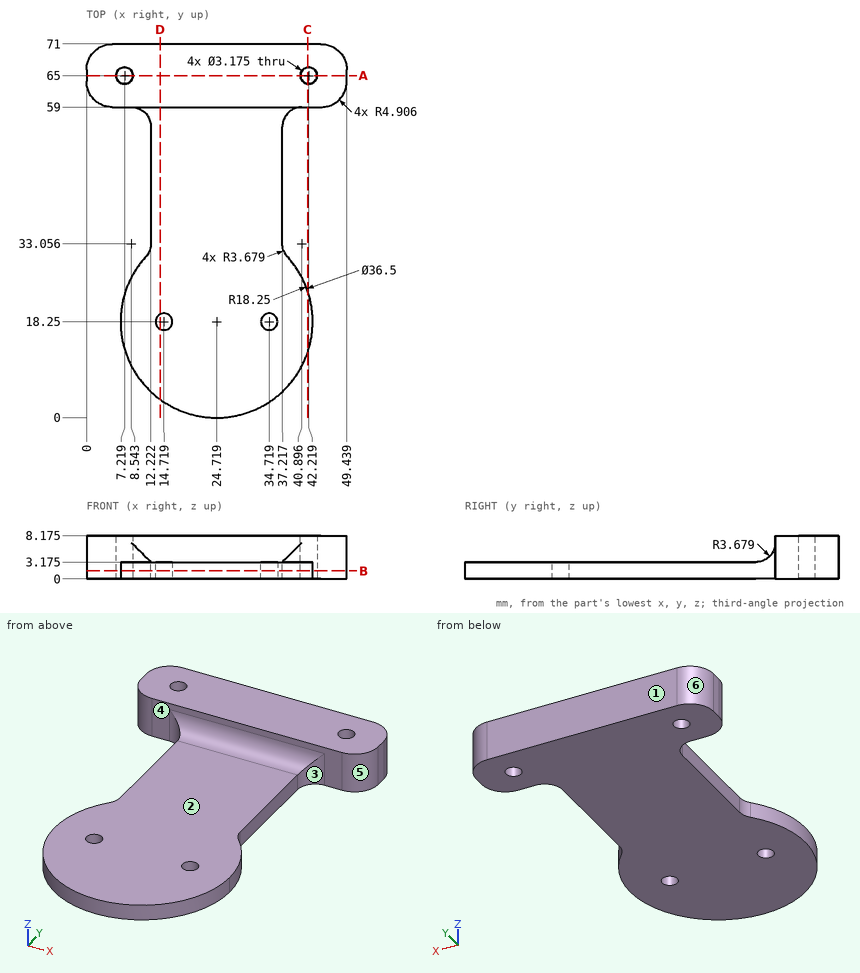
Here's the drawing with two shaded views (mm, measured from the low corner). I have some questions. A direction names the side the tool comes from. Round coordinates to 2 decimals unless told otherwise and drop trailing zeros. Loops run counter-clockwise (first coordinate to the right, second up) from the corner with the lowest first, then second, coordinate; pieces in that order, holes last. Notation, with made-up numbers: M -0.75,-12 L 25.25,-12 A15 ccw 25.25,16 Z; hole C -23.5,-35.5 d7. An arc over 180 degrees is marked long. Answer as a JSON object with one key per item and string values. Group by question number.
Q1. We'd pull the mould along Y, two halves only. Please class the marked faces 3, 4, 5 and 6: +Y half, -Y half, draft (parallel to the pull), parting line (faces both ways), or undercut.
Q2. Imagine slicing it at B-B, the plane z = 1.5. Count the separate pieces of the cut face and the enclosed holes in it, then the cut area to 3 significant figures.
Q3. Imagine slicing it at D-D, the plane x = 14. Please give me the cut outline in (y, z) (1 decimal).
Q4. Will these pins go through, and if not, where does the flat tip stop? pin 1 (3 mm diameter, centred on x = 42.22, y = 65, fed in from -Z); pin 2 (4 mm diameter, centred on y = 23.5, z = 4, fed in from -X); pin 3 (3.5 mm diameter, centred on x = 14.72, y = 18.25, fed in from +Z) (3 decimals); pin 4 (4 mm diameter, centred on x = 16, z = 3, fed in from -Y).
Q5. Please list where these lines run through material, in increasing order: L1, parallel to X at y = 18.25, z = 1.6; L2, parallel to X at y = 65, z = 4.75; L3, parallel to Y at x = 43.5, z = 2.75.
Q6. On a 3-axis mill with a long thin cutter (end or side, diameter ignored), from which of +Z, -Z, +X, -X, +Y, -Y can I reach the whole of each face in a straight line? I mean the marked faces 1 and 2. Say none if no direction works.
Q7. Imagine slicing it at C-C, the plane x = 42. Please give me the cut outline in (y, z) (1 decimal), then the cut area to 3 significant figures.
Q8. Imagine slicing it at A-A, the plane y = 65. Please give me the cut outline in (x, z) (1 decimal), then the cut area to 3 significant figures.
Findings:
{
 "1": {"face 3": "undercut", "face 4": "undercut", "face 5": "-Y half", "face 6": "+Y half"},
 "2": {"separate pieces": "1", "enclosed holes": "4", "area": "2,190 mm2"},
 "3": {"outline": "M 3.5,0 L 16.8,0 L 16.8,3.2 L 3.5,3.2 Z; M 19.7,0 L 71,0 L 71,8.2 L 59,8.2 L 59,6.9 A3.7 cw 55.3,3.2 L 19.7,3.2 Z"},
 "4": {"pin 1": "passes through", "pin 2": "stops at x = 6.79", "pin 3": "stops at z = 3.175", "pin 4": "stops at y = 1.28"},
 "5": {"L1": "x = 6.47 to 13.13, 16.31 to 33.13, 36.31 to 42.97", "L2": "x = 0 to 5.63, 8.81 to 40.63, 43.81 to 49.44", "L3": "y = 59 to 64.06, 65.94 to 71"},
 "6": {"face 1": "+Z, -Z, +X, -X, +Y", "face 2": "+Z, +X, -X, -Y"},
 "7": {"outline": "M 12.4,0 L 24.1,0 L 24.1,3.2 L 12.4,3.2 Z; M 59,0 L 63.4,0 L 63.4,8.2 L 59,8.2 Z; M 66.6,0 L 71,0 L 71,8.2 L 66.6,8.2 Z", "area": "110 mm2"},
 "8": {"outline": "M 0,0 L 5.6,0 L 5.6,8.2 L 0,8.2 Z; M 8.8,0 L 40.6,0 L 40.6,8.2 L 8.8,8.2 Z; M 43.8,0 L 49.4,0 L 49.4,8.2 L 43.8,8.2 Z", "area": "352 mm2"}
}
